from build123d import *

# Parameters (mm, degrees)
F0_R     = 3.175
F1_DEPTH = 19.05


with BuildPart() as f1:
    # F0 (on Front) → F1 (new body)
    with BuildSketch(Plane.XZ):
        with BuildLine():
            Line((-203.9060870256, -443.1007931722), (-197.1510368857, -432.7144915486))
            Line((-197.1510368857, -432.7144915486), (176.0463190104, 141.0992068278))
            ThreePointArc((176.0463190104, 141.0992068278), (170.463048361, 167.4550807244), (144.1071744644, 161.871810075))
            Line((144.1071744644, 161.871810075), (-235.8452315716, -422.328189925))
            ThreePointArc((-235.8452315716, -422.328189925), (-230.2619609222, -448.6840638216), (-203.9060870256, -443.1007931722))
        make_face()
        with Locations((-219.8756592986, -432.7144915486)):
            Circle(F0_R, mode=Mode.SUBTRACT)
        with Locations((160.0767467374, 151.4855084514)):
            Circle(F0_R, mode=Mode.SUBTRACT)
    extrude(amount=F1_DEPTH)


solid = f1.part
Can you work these out from the model? Positions are in its coordinate system, mm. Give positions to 0.01 mm unless a question says otherwise; leave off trailing zeros. Loops run counter-clockwise (first coordinate to the right, second up) from the corner with the lowest first, then second, coordinate; pieces in that order, holes last. Notation, with made-up numbers: (76, 58) -> (134, 58) arc R26 cw to (134, 74) -> close; hole circle Ø1 at (13, 16.5). An arc over 180 degrees is marked (long way). Use one line per item in the form item = value.
1) I need wall thicknesses on line 1 along Z through (x, y) = (73, -15); line 2 along X through (y, z) = (-1.75, -329.5); line 3 along X through (y, z) = (-13, -346.5). Which ranges of each line are inside material? Lowest first, please.
Answers:
line_1 = -17.34 to 52.54
line_2 = -175.47 to -130.02
line_3 = -186.53 to -141.08
2) Will these pins go through, and if not, where does the flat tip stop? pin 1 (3 mm diameter, centred on y = -11, z = -176, fed in from +X); pin 2 (6 mm diameter, centred on y = -14, z = 59, fed in from -X); pin 3 (8 mm diameter, centred on y = -3.5, z = -263, fed in from +X).
Answers:
pin_1 = -29.21
pin_2 = 75.25
pin_3 = -84.17
3) If we section it at C-C (x = 69): Please give me the cut outline in (y, z).
Answers:
outline = (-19.05, -23.49) -> (0, -23.49) -> (0, 46.39) -> (-19.05, 46.39) -> close
4) If we section it at A-A (y = -9.25): Count the separate pieces of the cut face and the enclosed holes in it, plus the area to 3 significant figures.
Answers:
separate_pieces = 1
enclosed_holes = 2
area = 27,600 mm²
5) If we section it at B-B (z = -130): Please give me the cut outline in (x, y), plus the area to 3 significant figures.
Answers:
outline = (-45.72, -19.05) -> (-0.27, -19.05) -> (-0.27, 0) -> (-45.72, 0) -> close
area = 866 mm²
